from build123d import *

# Parameters (mm, degrees)
F1_DEPTH = 5.5
F2_R     = 7
F3_DEPTH = 1
F4_R     = 2.5
F5_DEPTH = 12


with BuildPart() as f1:
    # F0 (on Front) → F1 (new body)
    with BuildSketch(Plane.XZ):
        Polygon((0, 4), (2.309401, 0), (6.928203, 0), (9.237604, 4), (6.928203, 8), (2.309401, 8), align=None)
    extrude(amount=F1_DEPTH)

    # F2 (on face) → F3 (join)
    with BuildSketch(Plane(origin=(0, 0, 0), x_dir=(-1, 0, 0), z_dir=(0, 1, 0))):
        with Locations((-4.618802, 4)):
            Circle(F2_R)
        Polygon((-2.309401, 8), (0, 4), (-2.309401, 0), (-6.928203, 0), (-9.237604, 4), (-6.928203, 8), align=None, mode=Mode.SUBTRACT)
    extrude(amount=-F3_DEPTH)

    # F4 (on face) → F5 (join)
    with BuildSketch(Plane(origin=(0, 0, 0), x_dir=(-1, 0, 0), z_dir=(0, 1, 0))):
        with Locations((-4.618802, 4)):
            Circle(F4_R)
    extrude(amount=F5_DEPTH)


solid = f1.part
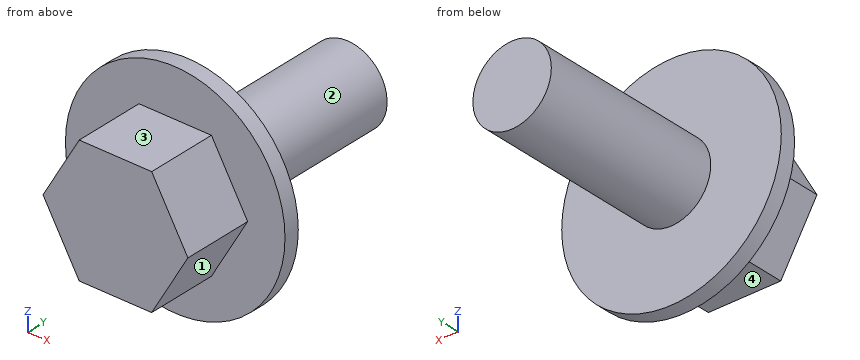
Could you check a few things on this model? Use its own coordinates, in mm. Face numbers are marked on the shaded views. A direction names the side the tool comes from. Coordinates: 2 decimals unless noted, no trailing zeros. Loops run counter-clockwise (first coordinate to the right, second up) from the corner with the lowest first, then second, coordinate; pieces in that order, holes last. Notation, with made-up numbers: (22.25, 43) -> (30.25, 43) arc R7 ccw to (30.25, 48) -> close; hole circle Ø2 at (73.25, 78). An arc over 180 degrees is marked (long way). Answer in a Markdown table with one row per item.
(1) Will these pins go through, and if not, where does the flat tip stop? pin 1 Ø5 at (y, z) = (8.5, 6.5) entering from +X; pin 2 Ø1.5 at (x, y) = (7.5, -1.5) entering from +Z; pin 3 Ø1.3 at (x, y) = (3.5, -4.5) entering from -Z.
Results found:
| item | result |
|---|---|
| pin 1 | stops at x = 7.12 |
| pin 2 | stops at z = 10.6 |
| pin 3 | stops at z = 0 |
(2) If I drill on probe 1 along Y at (x, z) = (9.25, 6.75); probe 2 along Z at (x, y) = (3.5, -4); probe 3 along Z at (x, y) = (4.5, 5), over which ranges is the centre line in solid material (lowest first)?
Results found:
| item | result |
|---|---|
| probe 1 | y = -1 to 0 |
| probe 2 | z = 0 to 8 |
| probe 3 | z = 1.5 to 6.5 |
(3) Imagine slicing it at C-C (y = -1.25). List the corners of the cut face in (x, z) for me, plus the area to 3 significant figures.
Results found:
| item | result |
|---|---|
| outline | (0, 4) -> (2.31, 0) -> (6.93, 0) -> (9.24, 4) -> (6.93, 8) -> (2.31, 8) -> close |
| area | 55.4 mm^2 |
(4) Imagine slicing it at B-B (z = 0.5). List the corners of the cut face in (x, y) for me.
Results found:
| item | result |
|---|---|
| outline | (-1.44, -1) -> (2.02, -1) -> (2.02, -5.5) -> (7.22, -5.5) -> (7.22, -1) -> (10.68, -1) -> (10.68, 0) -> (-1.44, 0) -> close |
(5) For the marked faces 1, 2, 3 and 4, which set-ups out of +Z, -Z, +X, -X, +Y, -Y let a thin tool reach every point of the face, with its end or its side?
Results found:
| item | result |
|---|---|
| face 1 | -Z, +X, -Y |
| face 2 | +Y |
| face 3 | +Z, +X, -X, -Y |
| face 4 | -Z, +X, -X, -Y |
(6) Imagine slicing it at A-A (x = 1.5). List the corners of the cut face in (y, z) for me.
Results found:
| item | result |
|---|---|
| outline | (-5.5, 1.4) -> (-1, 1.4) -> (-1, -2.27) -> (0, -2.27) -> (0, 10.27) -> (-1, 10.27) -> (-1, 6.6) -> (-5.5, 6.6) -> close |
(7) Imagine slicing it at D-D (x = 5.5). List the corners of the cut face in (y, z) for me.
Results found:
| item | result |
|---|---|
| outline | (-5.5, 0) -> (-1, 0) -> (-1, -2.94) -> (0, -2.94) -> (0, 1.66) -> (12, 1.66) -> (12, 6.34) -> (0, 6.34) -> (0, 10.94) -> (-1, 10.94) -> (-1, 8) -> (-5.5, 8) -> close |
